Check sheet for the modelled part. Datum: model origin and axes. Units: mm. A direction names the side the tool comes from. Give positions to 0.01 mm unless a question says otherwise; leave off trailing zeros. Order: outer loops, then holes, each group sorted by start corner. A loop starts at its lowest first (then second) coordinate and runs counter-clockwise, first axis right, second up.
from build123d import *

# Parameters (mm, degrees)
F0_W     = 150
F0_H     = 320
F0_R     = 56.5
F0_R_2   = 37
F1_DEPTH = 18
F2_DEPTH = 8
F3_DEPTH = 13
F4_DEPTH = 25
F5_DEPTH = 25


with BuildPart() as f1:
    # F0 (on Front) → F1 (new body)
    with BuildSketch(Plane.XZ):
        with Locations((51.2499984354, 41.7307654023)):
            Rectangle(F0_W, F0_H)
        with BuildLine():
            ThreePointArc((31.135600184, 99.7785914893), (22.4571929891, 191.0317394622), (103.2499984354, 147.7307654023))
            ThreePointArc((103.2499984354, 147.7307654023), (94.5509724953, 118.9379599561), (71.3643966867, 99.7785914893))
            ThreePointArc((71.3643966867, 99.7785914893), (107.4105178311, 74.5158831023), (121.2499984354, 32.7307654023))
            ThreePointArc((121.2499984354, 32.7307654023), (9.4648807354, -23.4297539934), (31.135600184, 99.7785914893))
        make_face(mode=Mode.SUBTRACT)
        with BuildLine():
            ThreePointArc((71.3643966867, 99.7785914893), (51.2499984354, 95.7307654023), (31.135600184, 99.7785914893))
            ThreePointArc((31.135600184, 99.7785914893), (9.4648807354, -23.4297539934), (121.2499984354, 32.7307654023))
            ThreePointArc((121.2499984354, 32.7307654023), (107.4105178311, 74.5158831023), (71.3643966867, 99.7785914893))
        make_face()
        with Locations((51.2499984354, 32.7307654023)):
            Circle(F0_R, mode=Mode.SUBTRACT)
        with Locations((51.2499984354, 32.7307654023)):
            Circle(F0_R)
        with BuildLine():
            ThreePointArc((71.3643966867, 99.7785914893), (94.5509724953, 118.9379599561), (103.2499984354, 147.7307654023))
            ThreePointArc((103.2499984354, 147.7307654023), (22.4571929891, 191.0317394622), (31.135600184, 99.7785914893))
            ThreePointArc((31.135600184, 99.7785914893), (51.2499984354, 102.7307654023), (71.3643966867, 99.7785914893))
        make_face()
        with Locations((51.2499984354, 147.7307654023)):
            Circle(F0_R_2, mode=Mode.SUBTRACT)
        with Locations((51.2499984354, 147.7307654023)):
            Circle(F0_R_2)
        with BuildLine():
            ThreePointArc((71.3643966867, 99.7785914893), (51.2499984354, 102.7307654023), (31.135600184, 99.7785914893))
            ThreePointArc((31.135600184, 99.7785914893), (51.2499984354, 95.7307654023), (71.3643966867, 99.7785914893))
        make_face()
    extrude(amount=F1_DEPTH)

    # F0 (on Front) → F2 (cut)
    with BuildSketch(Plane.XZ):
        with BuildLine():
            ThreePointArc((71.3643966867, 99.7785914893), (51.2499984354, 95.7307654023), (31.135600184, 99.7785914893))
            ThreePointArc((31.135600184, 99.7785914893), (9.4648807354, -23.4297539934), (121.2499984354, 32.7307654023))
            ThreePointArc((121.2499984354, 32.7307654023), (107.4105178311, 74.5158831023), (71.3643966867, 99.7785914893))
        make_face()
        with Locations((51.2499984354, 32.7307654023)):
            Circle(F0_R, mode=Mode.SUBTRACT)
        with Locations((51.2499984354, 32.7307654023)):
            Circle(F0_R)
        with BuildLine():
            ThreePointArc((71.3643966867, 99.7785914893), (51.2499984354, 102.7307654023), (31.135600184, 99.7785914893))
            ThreePointArc((31.135600184, 99.7785914893), (51.2499984354, 95.7307654023), (71.3643966867, 99.7785914893))
        make_face()
    extrude(amount=F2_DEPTH, mode=Mode.SUBTRACT)

    # F0 (on Front) → F3 (cut)
    with BuildSketch(Plane.XZ):
        with BuildLine():
            ThreePointArc((71.3643966867, 99.7785914893), (94.5509724953, 118.9379599561), (103.2499984354, 147.7307654023))
            ThreePointArc((103.2499984354, 147.7307654023), (22.4571929891, 191.0317394622), (31.135600184, 99.7785914893))
            ThreePointArc((31.135600184, 99.7785914893), (51.2499984354, 102.7307654023), (71.3643966867, 99.7785914893))
        make_face()
        with Locations((51.2499984354, 147.7307654023)):
            Circle(F0_R_2, mode=Mode.SUBTRACT)
        with Locations((51.2499984354, 147.7307654023)):
            Circle(F0_R_2)
        with BuildLine():
            ThreePointArc((71.3643966867, 99.7785914893), (51.2499984354, 102.7307654023), (31.135600184, 99.7785914893))
            ThreePointArc((31.135600184, 99.7785914893), (51.2499984354, 95.7307654023), (71.3643966867, 99.7785914893))
        make_face()
    extrude(amount=F3_DEPTH, mode=Mode.SUBTRACT)

    # F0 (on Front) → F4 (cut)
    with BuildSketch(Plane.XZ):
        with Locations((51.2499984354, 147.7307654023)):
            Circle(F0_R_2)
    extrude(amount=F4_DEPTH, mode=Mode.SUBTRACT)

    # F0 (on Front) → F5 (cut)
    with BuildSketch(Plane.XZ):
        with Locations((51.2499984354, 32.7307654023)):
            Circle(F0_R)
    extrude(amount=F5_DEPTH, mode=Mode.SUBTRACT)


solid = f1.part
1) Section check D-D, the plane y = -4. Record the cut outline in (x, z), then the cut area to 3 significant figures.
Recorded:
outline: (-23.75, -118.27) - (126.25, -118.27) - (126.25, 201.73) - (-23.75, 201.73) - close; hole (31.14, 99.78) arc R70 ccw (long way) to (71.36, 99.78) arc R52 ccw (long way) to start
area: 24,300 mm2
2) Section check C-C, the plane x = 68. Record the cut outline in (y, z), then the cut area to 3 significant figures.
Recorded:
outline: (-18, -118.27) - (0, -118.27) - (0, -35.24) - (-8, -35.24) - (-8, -21.23) - (-18, -21.23) - close; (-18, 86.69) - (-8, 86.69) - (-8, 98.5) - (-13, 98.5) - (-13, 114.74) - (-18, 114.74) - close; (-18, 180.72) - (-13, 180.72) - (-13, 196.96) - (0, 196.96) - (0, 201.73) - (-18, 201.73) - close
area: 2,000 mm2
3) Material ranges on L1, parallel to X at y = -8.5, z = 147.5; L2, parallel to Z at x = 81, y = -3.5; L3, parallel to Z at x = 24, y = -8.5, recorded low to high.
Recorded:
L1: x = -23.75 to -0.75, 103.25 to 126.25
L2: z = -118.27 to -30.63, 96.09 to 105.08, 190.38 to 201.73
L3: z = -118.27 to -16.76, 82.23 to 103.44, 192.02 to 201.73
4) Set-up check for faces 1 (the face through (16, -13, 160)), 2 (the face through (0, -18, 8)): record each of +Z, -Z, +X, -X, +Y, -Y from which the full face is reachable in a straight line by a thin tool's end or side.
Recorded:
face 1: +Y
face 2: +Z, -Z, +X, -X, -Y
5) Depth check by flat-ended pin: pin 1 Ø6 at (x, z) = (30, 115) entering from +Y; pin 2 Ø6 at (x, z) = (21.5, 137.5) entering from +Y. Enter the tip coordinate at first touch or a pass-through.
Recorded:
pin 1: stops at y = -13
pin 2: passes through
6) Draft check along Z on faces 3 (the face through (50, -9, 201.731)), 4 (the face through (68.83, -6.41, 196.67)), 5 (the face through (126.25, -9, 39)), 6 (the face through (50, -9, -118.269)). Enter one of: +Z half, -Z half, draft (parallel to the pull), parting line (faces both ways), or undercut.
Recorded:
face 3: +Z half
face 4: undercut
face 5: draft
face 6: -Z half
7) Section check A-A, the plane x = 98. Record the cut outline in (y, z), then the cut area to 3 significant figures.
Recorded:
outline: (-18, -118.27) - (0, -118.27) - (0, -19.37) - (-8, -19.37) - (-8, 1) - (-18, 1) - close; (-18, 64.46) - (-8, 64.46) - (-8, 84.83) - (0, 84.83) - (0, 124.96) - (-13, 124.96) - (-13, 170.5) - (0, 170.5) - (0, 201.73) - (-18, 201.73) - close
area: 3,700 mm2
8) Section check B-B, the plane z = 41. Record the cut outline in (x, y).
Recorded:
outline: (-23.75, -18) - (-4.64, -18) - (-4.64, -8) - (-18.26, -8) - (-18.26, 0) - (-23.75, 0) - close; (107.14, -18) - (126.25, -18) - (126.25, 0) - (120.76, 0) - (120.76, -8) - (107.14, -8) - close
